Verification items for the finished model (mm, model axes). Face numbers are marked on the shaded views. A direction names the side the tool comes from. Coordinates: 2 decimals unless noted, no trailing zeros. Write each loop counter-clockwise with the first axis right and the second up, starting at its lowest first coordinate (ties: lowest second). Pieces come first, ordered by that corner, then holes. Notation, with made-up numbers: (86, -21.5) -> (119, -21.5) arc R16 ccw to (119, 3.5) -> close; hole circle Ø5 at (53.25, 64.25). An arc over 180 degrees is marked (long way). Answer in a Markdown table with one row per item.
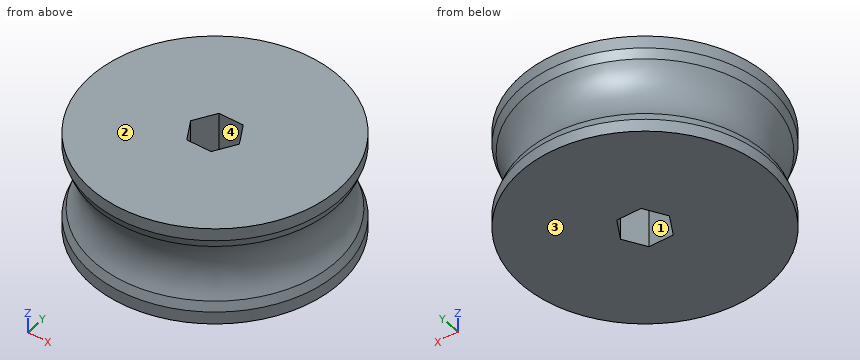
```python
from build123d import *

# Parameters (mm, degrees)
SKETCH1_R           = 25
BOSS_EXTRUDE1_DEPTH = 20
CUT_EXTRUDE1_DEPTH  = 41.620192023


with BuildPart() as part:
    # Sketch1 → Boss-Extrude1 (new body)
    with BuildSketch(Plane.XY):
        Circle(SKETCH1_R)
    extrude(amount=BOSS_EXTRUDE1_DEPTH)

    # Sketch2 → Cut-Revolve1 (revolve, cut)
    with BuildSketch(Plane(origin=(0, 0, 0), x_dir=(0, 0, -1), z_dir=(1, 0, 0)), mode=Mode.PRIVATE) as cut_revolve1_sk:
        with BuildLine():
            Line((-17.5, 25), (-15.75, 24.318465914))
            ThreePointArc((-15.75, 24.318465914), (-10, 22.5), (-4.25, 24.318465914))
            Line((-4.25, 24.318465914), (-2.5, 25))
            Line((-2.5, 25), (-17.5, 25))
        make_face()
    revolve(cut_revolve1_sk.sketch.rotate(Axis((0, 0, 20), (0, 0, -1)), 90), axis=Axis((0, 0, 20), (0, 0, -1)), mode=Mode.SUBTRACT)

    # Sketch3 → Cut-Extrude1 (cut, through all)
    with BuildSketch(Plane(origin=(0, 0, 0), x_dir=(-1, 0, 0), z_dir=(0, 0, -1))):
        Polygon((5, 0), (2.5, 4.330127019), (-2.5, 4.330127019), (-5, 0), (-2.5, -4.330127019), (2.5, -4.330127019), align=None)
    extrude(amount=-CUT_EXTRUDE1_DEPTH, mode=Mode.SUBTRACT)


solid = part.part
```
1. Tool access check on the marked faces 3 and 4. Record the directions out of +Z, -Z, +X, -X, +Y, -Y that give a thin tool (end or side, any length) a straight path to the whole face; none if there is none.
Geometry says:
| item | result |
|---|---|
| face 3 | -Z, +X, -X, +Y, -Y |
| face 4 | +Z, -Z |
2. Depth check by flat-ended pin: P1, Ø5, axis at x = -11.5, z = 14.5, coming from the -Y side; P2, Ø4, axis at x = 0.5, z = 13, coming from the -Y side; P3, Ø1.5, axis at x = -0.5, z = 13.5, coming from the +Y side. Enter the tip coordinate at first touch or a pass-through.
Geometry says:
| item | result |
|---|---|
| P1 | y = -22.51 |
| P2 | y = -23.84 |
| P3 | y = 23.44 |
3. Mould release check, pull along Y, two halves, no side actions. Record for the marked faces 1 and 2: released by +Y, released by -Y, zero draft, split by the parting line, or undercut.
Geometry says:
| item | result |
|---|---|
| face 1 | undercut |
| face 2 | zero draft |
4. Section check B-B, the plane z = 5. Record the boundary of the cut face in (x, y).
Geometry says:
| item | result |
|---|---|
| outline | circle Ø47.68 at (0, 0); hole (-5, 0) -> (-2.5, -4.33) -> (2.5, -4.33) -> (5, 0) -> (2.5, 4.33) -> (-2.5, 4.33) -> close |
5. Section check A-A, the plane x = 0. Record the boundary of the cut face in (y, z).
Geometry says:
| item | result |
|---|---|
| outline | (-25, 0) -> (-4.33, 0) -> (-4.33, 20) -> (-25, 20) -> (-25, 17.5) -> (-24.32, 15.75) arc R10 cw to (-24.32, 4.25) -> (-25, 2.5) -> close; (4.33, 0) -> (25, 0) -> (25, 2.5) -> (24.32, 4.25) arc R10 cw to (24.32, 15.75) -> (25, 17.5) -> (25, 20) -> (4.33, 20) -> close |
6. Section check C-C, the plane z = 14.25. Record the boundary of the cut face in (x, y).
Geometry says:
| item | result |
|---|---|
| outline | circle Ø46.9 at (0, 0); hole (-5, 0) -> (-2.5, -4.33) -> (2.5, -4.33) -> (5, 0) -> (2.5, 4.33) -> (-2.5, 4.33) -> close |
7. Thickness scan on line 1 (X direction, y = -4, z = 6); line 2 (Y direction, x = 14, z = 10.25); line 3 (X direction, y = 8.5, z = 10.5). Record the ranges inside material, lowest first. Write a range as from..to.
Geometry says:
| item | result |
|---|---|
| line 1 | -22.99..-2.69, 2.69..22.99 |
| line 2 | -17.62..17.62 |
| line 3 | -20.85..20.85 |
